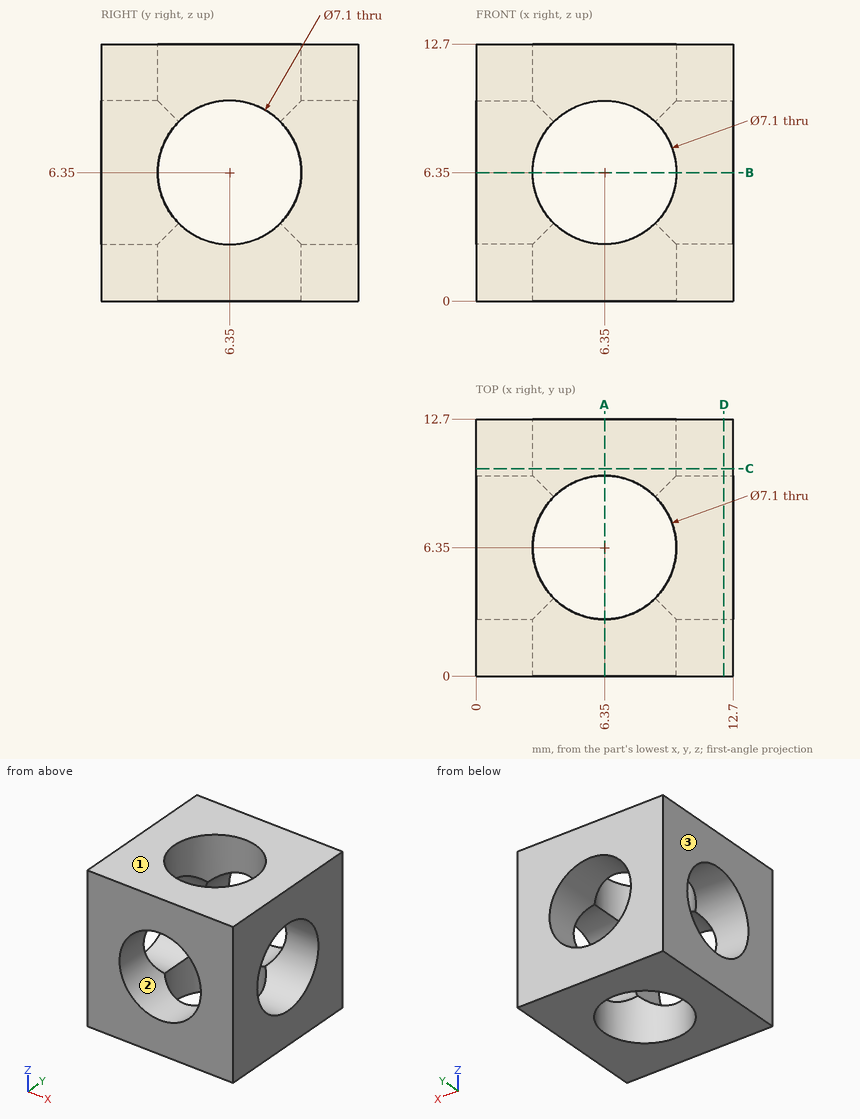
Source: three-view drawing plus pictorial views. Frame: mm from the lowest corner of the part. Give positions to 0.01 mm unless a question says otherwise; leave off trailing zeros. Order: outer loops, then holes, each group sorted by start corner. A loop starts at its lowest first (then second) coordinate and runs counter-clockwise, first axis right, second up.
1. Section A-A on x = 6.35. Return the cut outline in (y, z), and give its area (3 significant figures).
Derived:
outline: (0, 0) - (2.8, 0) - (2.8, 2.8) - (0, 2.8) - close; (0, 9.9) - (2.8, 9.9) - (2.8, 12.7) - (0, 12.7) - close; (9.9, 0) - (12.7, 0) - (12.7, 2.8) - (9.9, 2.8) - close; (9.9, 9.9) - (12.7, 9.9) - (12.7, 12.7) - (9.9, 12.7) - close
area: 31.4 mm2
2. Section C-C on y = 10.25. Return the cut outline in (x, z), and give its area (3 significant figures).
Derived:
outline: (0, 0) - (12.7, 0) - (12.7, 12.7) - (0, 12.7) - close; hole circle Ø7.1 at (6.35, 6.35)
area: 122 mm2
3. Mould query, pull axis Z, two halves, no side actions, for the marked faces 1, 2 and 3. Classes: released by +Z, released by -Z, zero draft, split by the parting line, or undercut.
Derived:
face 1: released by +Z
face 2: undercut
face 3: zero draft
4. Material intervals for L1, parallel to Z at x = 6.35, y = 1, sorted ascending.
Derived:
L1: z = 0 to 2.8, 9.9 to 12.7
